Here's how the part is built. I have some questions about the finished solid (model axes, mm). Give positions to 0.01 mm unless a question says otherwise; leave off trailing zeros. Write each loop counter-clockwise with the first axis right and the second up, starting at its lowest first coordinate (ties: lowest second). Pieces come first, ordered by that corner, then holes. Notation, with made-up numbers: (-15, 34.25) -> (19, 34.25) arc R19 cw to (19, 57.25) -> close; hole circle Ø10 at (6.25, 18). An arc over 180 degrees is marked (long way). Use one line per item in the form item = value.
Autodesk Inventor part; units mm, degrees
ref_plane "YZ Plane" through (0, 0, 0) normal (1, 0, 0) x (0, 1, 0)
ref_plane "XZ Plane" through (0, 0, 0) normal (0, 1, 0) x (-1, 0, 0)
ref_plane "XY Plane" through (0, 0, 0) normal (0, 0, 1) x (1, 0, 0)
sketch "Sketch1" plane through (0, 0, 0) normal (1, 0, 0) x (0, 1, 0)
  line L0 (-25, 50) -> (25, 50)
  line L1 (25, 50) -> (25, -50)
  line L2 (25, -50) -> (-25, -50)
  line L3 (-25, -50) -> (-25, 50)
  line L4 (-25, 50) -> (25, -50) construction
  line L5 (25, 50) -> (-25, -50) construction
  circle A0 centre (0, 40) radius 2.1
  circle A1 centre (0, 5) radius 2.1
  line L6 (0, 40) -> (0, 5)
  line L7 (25, 0) -> (-25, 0)
  circle A2 centre (0, -40) radius 2.1
  circle A3 centre (0, -5) radius 2.1
  point P0 (0, 0)
  point P1 (0, 50)
  dimension "d6" = 50
  dimension "d7" = 100
  dimension "d9" = 4.2
  dimension "d10" = 4.2
  dimension "d11" = 35
  dimension "d12" = 25
  dimension "d13" = 10
extrude "Extrusion2" add sketch "Sketch1" along normal blind 3
equation "\"d12\" = 0.5 * d6"
properties part number "motorPlate"
Q1. I want a section at B-B, the plane z = -5. Write out the boundary of the cut face in (x, y).
Result set:
outline = (0, -25) -> (3, -25) -> (3, -2.1) -> (0, -2.1) -> close; (0, 2.1) -> (3, 2.1) -> (3, 25) -> (0, 25) -> close
Q2. If we mould it in two halves opening along Y, with no side actions, what happens to faces 1 (the face through (1, -25, -1)), 2 (the face through (1.48, -0.46, -37.95)), 3 (the face through (1, 0, -50))? For each: +Y half, -Y half, draft (parallel to the pull), parting line (faces both ways), or undercut.
Result set:
face_1 = -Y half
face_2 = undercut
face_3 = draft
Q3. I want a section at A-A, the plane y = 0. Write out the boundary of the cut face in (x, z).
Result set:
outline = (0, -50) -> (3, -50) -> (3, -42.1) -> (0, -42.1) -> close; (0, -37.9) -> (3, -37.9) -> (3, -7.1) -> (0, -7.1) -> close; (0, -2.9) -> (3, -2.9) -> (3, 2.9) -> (0, 2.9) -> close; (0, 7.1) -> (3, 7.1) -> (3, 37.9) -> (0, 37.9) -> close; (0, 42.1) -> (3, 42.1) -> (3, 50) -> (0, 50) -> close
Q4. If I drill on line 1 along Z through (x, y) = (1.5, 0); line 2 along Y through (x, z) = (2.15, 40), over which ranges is the centre line in solid material (lowest first)? Write a range as from..to.
Result set:
line_1 = -50..-42.1, -37.9..-7.1, -2.9..2.9, 7.1..37.9, 42.1..50
line_2 = -25..-2.1, 2.1..25
